```python
from build123d import *

# Parameters (mm, degrees)
F1_DEPTH = 90
F2_T     = -2.5
F3_DEPTH = 6
F5_DEPTH = 50


with BuildPart() as f1:
    # F0 (on Front) → F1 (new body)
    with BuildSketch(Plane.XZ):
        with BuildLine():
            Line((-25, 0), (25, 0))
            ThreePointArc((25, 0), (0, 25), (-25, 0))
        make_face()
    extrude(amount=F1_DEPTH)

    # F2
    f2_openings = [f1.faces().sort_by_distance(p)[0] for p in [
        (0, -90, 10.61033),
    ]]
    offset(amount=F2_T, openings=f2_openings)

    # F1_face (on face) → F3 (join)
    with BuildSketch(Plane(origin=(0, 0, 10.61033), x_dir=(1, 0, 0), z_dir=(0, 1, 0))):
        with BuildLine():
            Line((25, 10.61033), (-25, 10.61033))
            ThreePointArc((-25, 10.61033), (0, -14.38967), (25, 10.61033))
        make_face()
    extrude(amount=F3_DEPTH)

    # F4 (on Right) → F5 (cut, symmetric)
    with BuildSketch(Plane.YZ):
        Polygon((6, 47.765567), (6, 9.95), (8, 11.104701), (8, 47.765567), align=None)
        Polygon((8, -11.104701), (6, -9.95), (6, -25.27874), (8, -25.27874), align=None)
    extrude(amount=F5_DEPTH, both=True, mode=Mode.SUBTRACT)


solid = f1.part
```
Design review of the part built by this model. Coordinates are the model's own, in mm. A direction names the side the tool comes from. Coordinates: 2 decimals unless noted, no trailing zeros. Order: outer loops, then holes, each group sorted by start corner. A loop starts at its lowest first (then second) coordinate and runs counter-clockwise, first axis right, second up.
1) Take a section at B-B, the plane y = -27.5. Give the boundary of the cut face in (x, z).
2) Wall thickness on line 1 along Y through (x, z) = (4, 17); line 2 along Z through (x, y) = (13, -53.5); line 3 along Z through (x, y) = (-7, -64): over which ranges is each line inside the solid? List them lowest first.
3) Take a section at A-A, the plane x = 0. Give the boundary of the cut face in (y, z).
4) Clearance check with flat-ended pins moving along their axes: pin 1 (3 mm diameter, centred on y = -60, z = 20.5, fed in from +X); pin 2 (12 mm diameter, centred on y = -5.5, z = 17.5, fed in from +X); pin 3 (1 mm diameter, centred on y = -26.5, z = 5.5, fed in from -X). State where each tip first meets the part, or that it passes through.
5) Mouldability with a two-part tool opening along X and no side actions: class faces 3 (the flat face through (0, -2.5, 10)), 4 (the cylindrical face through (-0.55, -42.672, 24.994)), 5 (the flat face through (0, 6, 10)) as +X half, -X half, draft (parallel to the pull), parting line (faces both ways), or undercut.
6) For faces 1 (the flat face through (0, -43, 0)), 2 (the cylindrical face through (0.46, -45.638, 22.495)), list the 3-axis set-ups (+Z, -Z, +X, -X, +Y, -Y) from which the entire face can be reached by the end or side of a thin tool; tool diameter is ignored.
7) Take a section at C-C, the plane z = 15.5. Give the boundary of the cut face in (x, y), and give its area (3 significant figures).
Returned:
1. outline: (-25, 0) - (25, 0) arc R25 ccw to start; hole (-22.36, 2.5) - (22.36, 2.5) arc R22.5 ccw to start
2. line 1: y = -2.5 to 6
2. line 2: z = 0 to 2.5, 18.36 to 21.35
2. line 3: z = 0 to 2.5, 21.38 to 24
3. outline: (-90, 0) - (6, 0) - (6, 25) - (-90, 25) - (-90, 22.5) - (-2.5, 22.5) - (-2.5, 2.5) - (-90, 2.5) - close
4. pin 1: stops at x = 16.25
4. pin 2: stops at x = 22.2
4. pin 3: stops at x = -24.49
5. face 3: undercut
5. face 4: parting line
5. face 5: draft
6. face 1: -Z, +X, -X, +Y, -Y
6. face 2: -Y
7. outline: (-19.62, -90) - (-16.31, -90) - (-16.31, -2.5) - (16.31, -2.5) - (16.31, -90) - (19.62, -90) - (19.62, 6) - (-19.62, 6) - close
7. area: 912 mm2
